from build123d import *

# Parameters (mm, degrees)
SKETCH1_R           = 10
BOSS_EXTRUDE1_DEPTH = 25
FILLET2_R           = 0.5
FILLET3_R           = 0.5
SKETCH2_R           = 4
CUT_EXTRUDE1_DEPTH  = 12.5
SKETCH3_R           = 2.5
CUT_EXTRUDE2_DEPTH  = 12.5


with BuildPart() as part:
    # Sketch1 → Boss-Extrude1 (new body)
    with BuildSketch(Plane(origin=(0, 0, 0), x_dir=(1, 0, 0), z_dir=(0, 1, 0))):
        with Locations(Location((0, 0, 0), (0, 0, 270))):
            Circle(SKETCH1_R)
    extrude(amount=BOSS_EXTRUDE1_DEPTH)

    # Fillet2
    fillet2_edges = [part.edges().sort_by_distance(p)[0] for p in [
        (0, 25, -10),
    ]]
    fillet(fillet2_edges, radius=FILLET2_R)

    # Fillet3
    fillet3_edges = [part.edges().sort_by_distance(p)[0] for p in [
        (0, 0, -10),
    ]]
    fillet(fillet3_edges, radius=FILLET3_R)

    # Sketch2 → Cut-Extrude1 (cut)
    with BuildSketch(Plane.XZ):
        with Locations(Location((0, 0, 0), (0, 0, 270))):
            Circle(SKETCH2_R)
    extrude(amount=-CUT_EXTRUDE1_DEPTH, mode=Mode.SUBTRACT)

    # Sketch3 → Cut-Extrude2 (cut)
    with BuildSketch(Plane(origin=(0, 25, 0), x_dir=(1, 0, 0), z_dir=(0, 1, 0))):
        with Locations(Location((0, 0, 0), (0, 0, 270))):
            Circle(SKETCH3_R)
    extrude(amount=-CUT_EXTRUDE2_DEPTH, mode=Mode.SUBTRACT)


solid = part.part
Work out the finished part from the listing and answer in its coordinate system (mm). A direction names the side the tool comes from. Give positions to 0.01 mm unless a question says otherwise; leave off trailing zeros. Loops run counter-clockwise (first coordinate to the right, second up) from the corner with the lowest first, then second, coordinate; pieces in that order, holes last. Notation, with made-up numbers: (14.25, 44.25) - (22.25, 44.25) arc R11 ccw to (22.25, 59.25) - close; hole circle Ø2 at (76.5, 0). An arc over 180 degrees is marked (long way). Answer in a Markdown table with one row per item.
(1) Section B-B (z = 0) is taken. Give the vertices of the cut face in (x, y), and give its area (3 significant figures).
Results list:
| item | result |
|---|---|
| outline | (-10, 0.5) arc R0.5 ccw to (-9.5, 0) - (-4, 0) - (-4, 12.5) - (-2.5, 12.5) - (-2.5, 25) - (-9.5, 25) arc R0.5 ccw to (-10, 24.5) - close; (2.5, 12.5) - (4, 12.5) - (4, 0) - (9.5, 0) arc R0.5 ccw to (10, 0.5) - (10, 24.5) arc R0.5 ccw to (9.5, 25) - (2.5, 25) - close |
| area | 337 mm² |
(2) Section C-C (y = 1.75) is taken. Give the vertices of the cut face in (x, z).
Results list:
| item | result |
|---|---|
| outline | circle Ø20 at (0, 0); hole circle Ø8 at (0, 0) |
(3) Flat-ended cylindrical pins translate along their axes: pin 1 Ø2 at (y, z) = (16, 2.5) entering from -X; pin 2 Ø1.5 at (y, z) = (4, 6.5) entering from +X; pin 3 Ø10 at (x, y) = (6.5, 4) entering from -Z; pin 4 Ø3 at (x, z) = (0, 0) entering from -Y (1 decimal). Find the tip coordinate at first contact, or state that the pin passes through.
Results list:
| item | result |
|---|---|
| pin 1 | stops at x = -9.89 |
| pin 2 | stops at x = 8.18 |
| pin 3 | stops at z = -9.89 |
| pin 4 | passes through |
(4) Section D-D (y = 15.75) is taken. Give the vertices of the cut face in (x, z), and give its area (3 significant figures).
Results list:
| item | result |
|---|---|
| outline | circle Ø20 at (0, 0); hole circle Ø5 at (0, 0) |
| area | 295 mm² |
(5) For a pull along X with two mould halves and no side action, classify faces 1 (the face through (2, 12.5, -2)), 2 (the face through (-2, 25, 2)), 3 (the face through (-9.76, 12.33, -2.17)) as pulls with the +X half, pulls with the -X half, needs draft (parallel to the pull), parting line crosses it, or undercut.
Results list:
| item | result |
|---|---|
| face 1 | undercut |
| face 2 | needs draft |
| face 3 | parting line crosses it |
(6) Section A-A (x = 0) is taken. Give the vertices of the cut face in (y, z).
Results list:
| item | result |
|---|---|
| outline | (0, -9.5) arc R0.5 ccw to (0.5, -10) - (24.5, -10) arc R0.5 ccw to (25, -9.5) - (25, -2.5) - (12.5, -2.5) - (12.5, -4) - (0, -4) - close; (0, 4) - (12.5, 4) - (12.5, 2.5) - (25, 2.5) - (25, 9.5) arc R0.5 ccw to (24.5, 10) - (0.5, 10) arc R0.5 ccw to (0, 9.5) - close |
(7) Consider L1, parallel to X at y = 9.25, z = 0; L2, parallel to Y at x = -0.25, z = -2.75; L3, parallel to Z at x = -1.5, y = 19.5. Determine where each line is inside the solid, lowest interval first. Write a range as [from, to].
Results list:
| item | result |
|---|---|
| L1 | x = [-10, -4], [4, 10] |
| L2 | y = [12.5, 25] |
| L3 | z = [-9.89, -2], [2, 9.89] |
(8) A tool of negligible diameter and unlimited length cuts with its end or side. For faces 4 (the face through (-4, 0, 2)), 5 (the face through (-3.905, 6.162, 0.867)), from which of +Z, -Z, +X, -X, +Y, -Y can it reach the whole face along a straight path? Write none if from no direction.
Results list:
| item | result |
|---|---|
| face 4 | +Z, -Z, +X, -X, -Y |
| face 5 | -Y |
